from build123d import *

# Parameters (mm, degrees)
SKETCH1_R           = 40
SKETCH1_R_2         = 9.475
BOSS_EXTRUDE1_DEPTH = 24
FILLET1_R           = 12
SKETCH2_R           = 10.815
CUT_EXTRUDE1_DEPTH  = 5.08
CUT_EXTRUDE2_START  = -5.08
SKETCH3_R           = 10.815
CUT_EXTRUDE2_DEPTH  = 5.08


with BuildPart() as part:
    # Sketch1 → Boss-Extrude1 (new body)
    with BuildSketch(Plane(origin=(0, 0, 0), x_dir=(0, 0, -1), z_dir=(1, 0, 0))):
        Circle(SKETCH1_R)
        Circle(SKETCH1_R_2, mode=Mode.SUBTRACT)
    extrude(amount=BOSS_EXTRUDE1_DEPTH)

    # Fillet1
    fillet1_edges = [part.edges().sort_by_distance(p)[0] for p in [
        (0, 0, 40),
        (24, 0, 40),
    ]]
    fillet(fillet1_edges, radius=FILLET1_R - 0.0001)  # a hair under: the kernel refuses the full size

    # Sketch2 → Cut-Extrude1 (cut)
    with BuildSketch(Plane(origin=(24, 0, 0), x_dir=(0, 0, -1), z_dir=(1, 0, 0))):
        Circle(SKETCH2_R)
    extrude(amount=-CUT_EXTRUDE1_DEPTH, mode=Mode.SUBTRACT)

    # Sketch3 → Cut-Extrude2 (cut)
    with BuildSketch(Plane.ZY.offset(CUT_EXTRUDE2_START)):
        with Locations(Location((0, 0, 0), (0, 0, 180))):
            Circle(SKETCH3_R)
    extrude(amount=CUT_EXTRUDE2_DEPTH, mode=Mode.SUBTRACT)


solid = part.part
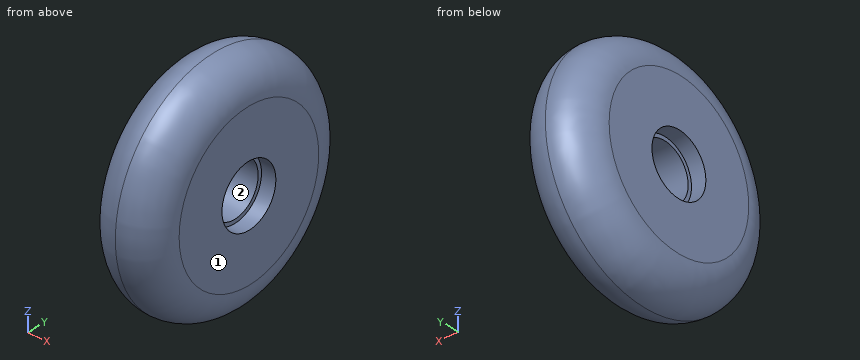
Check sheet for the modelled part. Datum: model origin and axes. Units: mm. Face numbers are marked on the shaded views. Give positions to 0.01 mm unless a question says otherwise; leave off trailing zeros. Write each loop counter-clockwise with the first axis right and the second up, starting at its lowest first coordinate (ties: lowest second). Pieces come first, ordered by that corner, then holes. Notation, with made-up numbers: (-17, 54) -> (-6, 54) arc R15 ccw to (-6, 59) -> close; hole circle Ø4 at (53.25, 36.5). An arc over 180 degrees is marked (long way). Use one line per item in the form item = value. Start each with the question number.
1. Section check D-D (x = 21.5). Record the cut outline in (y, z) (1 decimal).
2. Mould release check, pull along Y, two halves, no side actions. Record for the marked faces 1 and 2: pulls with the +Y half, pulls with the -Y half, needs draft (parallel to the pull), parting line crosses it, or undercut.
3. Section check C-C (x = 15.5). Record the cut outline in (y, z) (3 decimals).
4. Go/stop test with flat-tipped pins: P1, Ø17, axis at y = 0, z = 0, coming from the -X side; P2, Ø8, axis at x = 4.5, z = -10, coming from the +Y side; P3, Ø10, axis at x = 21, y = 19.5, coming from the -Z side; P4, Ø1, axis at x = 8, z = -12.5, coming from the -Y side. Record where each tip stops, or that it passes through.
5. Thickness scan on line 1 along Y through (x, z) = (22.5, 0) (3 decimals); line 2 along Y through (x, z) = (3, 0) (3 decimals); line 3 along Z through (x, y) = (6.5, -5.5). Record the ranges inside material, lowest first. Write a range as from..to.
Conclusion:
q1.outline = circle Ø70.7 at (0, 0); hole circle Ø21.6 at (0, 0)
q2.face_1 = needs draft
q2.face_2 = undercut
q3.outline = circle Ø78.957 at (0, 0); hole circle Ø18.95 at (0, 0)
q4.P1 = through
q4.P2 = 38.48
q4.P3 = -35.25
q4.P4 = -37.52
q5.line_1 = -33.81..-10.815, 10.815..33.81
q5.line_2 = -35.937..-10.815, 10.815..35.937
q5.line_3 = -38.27..-7.72, 7.72..38.27
